Autodesk Inventor part; units mm, degrees
ref_plane "YZ Plane" through (0, 0, 0) normal (1, 0, 0) x (0, 1, 0)
ref_plane "XZ Plane" through (0, 0, 0) normal (0, 1, 0) x (-1, 0, 0)
ref_plane "XY Plane" through (0, 0, 0) normal (0, 0, 1) x (1, 0, 0)
sketch "Sketch1" plane through (0, 0, 0) normal (0, 1, 0) x (-1, 0, 0)
  line L0 (0, 96.3881) -> (0, -80.6119)
  line L1 (0, -80.6119) -> (7.6619, -80.6119)
  line L2 (7.6619, -80.6119) -> (7.6619, -63.0119)
  line L3 (7.6619, -63.0119) -> (55.6286, -47.1119)
  line L4 (55.6286, -47.1119) -> (55.6286, 62.8881)
  line L5 (55.6286, 62.8881) -> (7.6619, 78.7881)
  line L6 (7.6619, 78.7881) -> (7.6619, 96.3881)
  line L7 (7.6619, 96.3881) -> (0, 96.3881)
  point P0 (0, 0)
  dimension "d0" = 177
  dimension "d1" = 17.6
  dimension "d2" = 17.6
  dimension "d3" = 110
  dimension "d4" = 15.9
extrude "Extrusion1" add sketch "Sketch1" along normal blind 150
sketch "Sketch2" plane through (0, 150, 0) normal (0, 1, 0) x (1, 0, 0)
  line L0 (-7.6619, -78.7881) -> (-7.6619, -96.3881)
  line L1 (-7.6619, -78.7881) -> (0, -78.7881)
  line L2 (0, -96.3881) -> (0, 80.6119)
  line L3 (0, -78.7881) -> (0, -67.7881)
  line L4 (0, -67.7881) -> (-7.6619, -67.7881)
  line L5 (-7.6619, 80.6119) -> (-7.6619, 63.0119)
  line L6 (-7.6619, 63.0119) -> (0, 63.0119)
  line L7 (0, 63.0119) -> (0, 52.0119)
  line L8 (0, 52.0119) -> (-7.6619, 52.0119)
  line L9 (0, -67.7881) -> (0, 52.0119)
  line L10 (-7.6619, -67.7881) -> (-47.625, -54.5411)
  line L11 (-7.6619, 52.0119) -> (-47.625, 38.7649)
  line L12 (-55.6286, -62.8881) -> (-7.6619, -78.7881)
  line L13 (-7.6619, 63.0119) -> (-55.6286, 47.1119)
  line L14 (-47.625, -54.5411) -> (-47.625, 38.7649)
  point P0 (0, 0)
  dimension "d8" = 11
  dimension "d9" = 11
  dimension "d10" = 0
  dimension "d11" = 0
  dimension "d12" = 93.306
extrude "Extrusion2" cut sketch "Sketch2" against normal blind 150
sketch "Sketch3" plane through (0, 0, -80.6119) normal (0, 0, -1) x (-1, 0, 0)
  line L0 (0, 0) -> (0, 150)
  line L1 (0, 135) -> (7.7027, 135)
  line L2 (7.7027, 135) -> (47.625, 122.3)
  line L3 (47.625, 150) -> (47.625, 0)
  line L4 (47.625, 122.3) -> (47.625, 101.6779)
  line L5 (47.625, 101.6779) -> (7.6619, 88.9625)
  line L6 (7.6619, 150) -> (7.6619, 0)
  line L7 (7.6619, 88.9625) -> (0, 88.9625)
  line L8 (0, 135) -> (0, 88.9625)
  line L9 (0, 73.9625) -> (7.7027, 73.9625)
  line L10 (7.7027, 73.9625) -> (47.625, 61.2625)
  line L11 (47.625, 61.2625) -> (47.625, 27.7154)
  line L12 (47.625, 27.7154) -> (7.6619, 15)
  line L13 (7.6619, 15) -> (0, 15)
  line L14 (0, 73.9625) -> (0, 15)
  line L15 (0, 150) -> (7.6619, 150)
  line L16 (0, 0) -> (7.6619, 0)
  point P0 (7.6619, 15)
  point P1 (7.6619, 73.9625)
  point P2 (7.6619, 135)
  dimension "d15" = 72.35
  dimension "d16" = 72.353
  dimension "d18" = 15
  dimension "d19" = 15
  dimension "d20" = 46.0375
  dimension "d22" = 72.353
  dimension "d23" = 72.35
  dimension "d24" = 15
extrude "Extrusion3" cut sketch "Sketch3" against normal blind 1500 contours L6 L9 L10 L3 L12 | L6 L1 L2 L3 L5
fillet "Fillet1" radius 2 8 edges at (-47.625, 122.3, -44.2649) (-47.625, 101.6779, -44.2649) (-47.625, 61.2625, -44.2649) (-47.625, 27.7154, -44.2649) (-47.625, 61.2625, 60.0411) (-47.625, 122.3, 60.0411) (-47.625, 101.6779, 60.0411) (-47.625, 27.7154, 60.0411)
fillet "Fillet2" radius 2 12 edges at (-47.625, 121.5687, 54.5411) (-47.625, 136.15, 54.5411) (-47.625, 60.5312, 54.5411) (-47.625, 102.4092, 54.5411) (-47.625, 28.4467, 54.5411) (-47.625, 13.8577, 54.5411) (-47.625, 136.15, -38.7649) (-47.625, 121.5687, -38.7649) (-47.625, 60.5312, -38.7649) (-47.625, 102.4092, -38.7649) (-47.625, 13.8577, -38.7649) (-47.625, 28.4467, -38.7649)
fillet "Fillet3" radius 2 4 edges at (-7.6619, 75, 96.3881) (-7.6619, 75, -80.6119) (-55.6286, 75, -47.1119) (-55.6286, 75, 62.8881)
sketch "Sketch4" plane through (-7.6619, 15, -52.0119) normal (-1, 0, 0) x (0, 0, 1)
  line L0 (130.8, 135) -> (146.4, 135)
  line L1 (139.9, 135) -> (139.9, -14.5366)
  line L2 (-20.1, 135) -> (-20.1, -15)
  line L3 (-26.6, -15) -> (-26.6, 135)
  line L4 (-26.6, -15) -> (-11, -15)
  line L5 (148.4, -15) -> (148.4, 135)
  circle A0 centre (-20.1, 127.5) radius 2.475
  line L6 (-26.6, 135) -> (-11, 135)
  circle A1 centre (-20.1, 66.4625) radius 2.475
  circle A2 centre (-20.1, -7.5) radius 2.475
  line L7 (-10.9865, 58.9625) -> (0.0135, 58.9625)
  point P0 (52.0119, -15)
  dimension "d30" = 160
  dimension "d31" = 150
  dimension "d32" = 0
  dimension "d33" = 8.5
  dimension "d34" = 4.95
  dimension "d35" = 7.5
  dimension "d36" = 7.5
  dimension "d37" = 7.5
extrude "Extrusion4" cut sketch "Sketch4" against normal blind 1500 contours A0 L2 | L2 A0 | A1 L2 | L2 A1 | A2 L2 | L2 A2
ref_plane "Work Plane1" through (-221.551, 135, 7.8881) normal (0, 0, -1) x (0, -1, 0)
mirror "Mirror1" about plane through (-221.551, 135, 7.8881) normal (0, 0, -1) of "Extrusion4"
sketch "Sketch5" plane through (-55.6286, 0, -45.6678) normal (-1, 0, 0) x (0, 0, 1)
  line L0 (99.426, 7.686) -> (7.686, 7.686)
  line L1 (7.686, 7.686) -> (7.686, 65.906)
  line L2 (7.686, 65.906) -> (99.426, 65.906)
  line L3 (99.426, 65.906) -> (99.426, 7.686)
  line L4 (0, 0) -> (0, 150)
  line L5 (0, 0) -> (107.1119, 0)
  circle A0 centre (29.446, 35.966) radius 3.5498
  circle A1 centre (84.636, 35.966) radius 3.8886
  point P0 (45.6678, 0)
  dimension "d40" = 58.22
  dimension "d41" = 91.74
  dimension "d42" = 7.686
  dimension "d43" = 7.686
  dimension "d44" = 21.76
  dimension "d45" = 29.94
  dimension "d46" = 55.19
  dimension "d47" = 29.94
extrude "Extrusion5" cut sketch "Sketch5" against normal blind 21.76 contours A0 | A1
equation "\"d48\" = d44"
properties part number "PiSpotAttachment"
Read the model definition and answer for the solid it produces. Units are mm, in the model's axes. A direction names the side the tool comes from. Round coordinates to 2 decimals unless told otherwise and drop trailing zeros. Write each loop counter-clockwise with the first axis right and the second up, starting at its lowest first coordinate (ties: lowest second). Pieces come first, ordered by that corner, then holes. Notation, with made-up numbers: (33, 3.5) -> (57, 3.5) arc R16 cw to (57, 9.5) -> close; hole circle Ø8 at (62, 43). An arc over 180 degrees is marked (long way). Answer in a Markdown table with one row per item. Add a question column.
1) Find section D-D, the plane y = 7.5. Determine the outline of the cut face in (x, z) (3 decimals), and give its area (3 significant figures).
2) Determine the mould class of faces 1 (the face through (-27.217, 21.222, -51.286)), 2 (the face through (-4, 76, -52.012)), 3 (the face through (-36.46, 73.95, 69.24)) for opening direction Z: pulls with the +Z half, pulls with the -Z half, needs draft (parallel to the pull), parting line crosses it, or undercut.
3) Consider line 1 (Z direction, x = -4, y = 77.5); line 2 (Z direction, x = -1.5, y = 142.5); line 3 (Y direction, x = -6.5, z = -71.5). Determine where each line is inside the solid, lowest interval first.
4) Given P1, Ø21.5, axis at y = 101, z = -67.5, coming from the -X side; P2, Ø4, axis at x = -11.5, y = 84.5, coming from the -Z side; P3, Ø12, axis at y = 64.5, z = 5, coming from the +X side (3 decimals), each flat-ended and moving along its own axis, determine where each tip first touches the part or whether it passes through.
5) Find section A-A, the plane y = 113.5. Determine the outline of the cut face in (x, z) (3 decimals).
6) Which of the six approach directions +Z, -Z, +X, -X, +Y, -Y give full straight-line access (tool end or side, diameter ignored) to faces 4 (the face through (-26.7, 139.6, -45.7)), 5 (the face through (-26.7, 67.92, 66.72)), 6 (the face through (-35.81, 73.95, -53.68))?
7) Find section B-B, the plane x = -12.5. Determine the outline of the cut face in (y, z).
8) Find section C-C, the plane z = 58.5. Determine the outline of the cut face in (x, y) (3 decimals), and give its area (3 significant figures).
Findings below:
| question | item | result |
|---|---|---|
| 1 | outline | (-55.629, -45.668) arc R2 ccw to (-54.258, -47.566) -> (-7.662, -63.012) -> (-7.662, -69.637) -> (0, -69.637) -> (0, -52.012) -> (-7.662, -52.012) -> (-46.254, -39.219) arc R2 cw to (-47.625, -37.321) -> (-47.625, 53.097) arc R2 cw to (-46.254, 54.995) -> (-7.662, 67.788) -> (0, 67.788) -> (0, 85.413) -> (-7.662, 85.413) -> (-7.662, 78.788) -> (-54.258, 63.342) arc R2 ccw to (-55.629, 61.444) -> close; (-7.662, -78.612) arc R2 ccw to (-5.662, -80.612) -> (0, -80.612) -> (0, -74.587) -> (-7.662, -74.587) -> close; (-7.662, 90.363) -> (0, 90.363) -> (0, 96.388) -> (-5.662, 96.388) arc R2 ccw to (-7.662, 94.388) -> close |
| 1 | area | 2,140 mm² |
| 2 | face 1 | needs draft |
| 2 | face 2 | undercut |
| 2 | face 3 | pulls with the +Z half |
| 3 | line 1 | -80.61 to -52.01, 67.79 to 96.39 |
| 3 | line 2 | -80.61 to -74.59, -69.64 to -52.01, 67.79 to 85.41, 90.36 to 96.39 |
| 3 | line 3 | 0 to 5.1, 9.9 to 79.06, 83.86 to 140.1, 144.9 to 150 |
| 4 | P1 | x = -7.66 |
| 4 | P2 | z = -62.4 |
| 4 | P3 | x = -47.625 |
| 5 | outline | (-55.629, -45.668) arc R2 ccw to (-54.258, -47.566) -> (-47.625, -49.765) -> (-47.625, 65.541) -> (-54.258, 63.342) arc R2 ccw to (-55.629, 61.444) -> close; (-7.662, -78.612) arc R2 ccw to (-5.662, -80.612) -> (0, -80.612) -> (0, -52.012) -> (-7.662, -52.012) -> close; (-7.662, 67.788) -> (0, 67.788) -> (0, 96.388) -> (-5.662, 96.388) arc R2 ccw to (-7.662, 94.388) -> close |
| 6 | face 4 | +X, +Y, -Y |
| 6 | face 5 | +Z, -Z |
| 6 | face 6 | -Z, -X, +Y, -Y |
| 7 | outline | (0, -61.41) -> (16.54, -61.41) -> (16.54, -50.41) -> (0, -50.41) -> close; (0, 66.18) -> (16.54, 66.18) -> (16.54, 77.18) -> (0, 77.18) -> close; (72.44, -61.41) -> (90.5, -61.41) -> (90.5, -50.41) -> (72.44, -50.41) -> close; (72.44, 66.18) -> (90.5, 66.18) -> (90.5, 77.18) -> (72.44, 77.18) -> close; (133.47, -61.41) -> (150, -61.41) -> (150, -50.41) -> (133.47, -50.41) -> close; (133.47, 66.18) -> (150, 66.18) -> (150, 77.18) -> (133.47, 77.18) -> close |
| 8 | outline | (-55.629, 0) -> (-35.682, 0) -> (-35.682, 23.915) -> (-46.231, 27.272) arc R2 cw to (-47.625, 29.178) -> (-47.625, 59.8) arc R2 cw to (-46.231, 61.706) -> (-35.682, 65.062) -> (-35.682, 97.878) -> (-46.231, 101.234) arc R2 cw to (-47.625, 103.14) -> (-47.625, 120.837) arc R2 cw to (-46.231, 122.743) -> (-35.682, 126.099) -> (-35.682, 150) -> (-55.629, 150) -> close |
| 8 | area | 2,260 mm² |
